Verification items for the finished model (mm, model axes). Round coordinates to 2 decimals unless told otherwise and drop trailing zeros. Write each loop counter-clockwise with the first axis right and the second up, starting at its lowest first coordinate (ties: lowest second). Pieces come first, ordered by that corner, then holes. Notation, with made-up numbers: (-39, 71.25) - (5, 71.25) arc R10 cw to (5, 76.25) - close; hole circle Ø5 at (59, 0.25). An arc over 180 degrees is marked (long way). Answer as a JSON object with one key per item and string values. Group by question number.
1) Section check A-A (x = 27). Enter the section's corners in (y, z) (3 decimals), then the cut area to 3 significant figures.
2) Thickness scan on line 1 (Z direction, x = 36.5, y = 0.25); line 2 (Z direction, x = 5, y = 0.3); line 3 (X direction, y = 0.1, z = -78). Record the ranges inside material, lowest first.
3) Mould release check, pull along Z, two halves, no side actions. Record for faces 1 (the flat face through (20, 0.675, -76)), 2 (the cylindrical face through (3.93, 0.34, -78.54)): +Z half, -Z half, draft (parallel to the pull), parting line (faces both ways), or undercut.
4) Section check C-C (z = -78.5). Enter the section's corners in (x, y) (3 decimals).
5) Section check B-B (y = 0.2). Enter the section's corners in (x, z).
```python
from build123d import *

# Parameters (mm, degrees)
SKETCH1_W           = 35
SKETCH1_H           = 12.964307825
BOSS_EXTRUDE1_DEPTH = 0.675
CUT_EXTRUDE1_DEPTH  = 0.68


with BuildPart() as part:
    # Sketch1 → Boss-Extrude1 (new body)
    with BuildSketch(Plane(origin=(0, 0, 0), x_dir=(1, 0, 0), z_dir=(0, 1, 0))):
        with Locations((19.821319384, 77.80811632)):
            Rectangle(SKETCH1_W, SKETCH1_H)
    extrude(amount=BOSS_EXTRUDE1_DEPTH)

    # Sketch2 → Cut-Extrude1 (cut)
    with BuildSketch(Plane(origin=(0, 0.675, 0), x_dir=(1, 0, 0), z_dir=(0, 1, 0))):
        with BuildLine():
            Line((13.502454123, 76.768011208), (37.321319384, 76.768011208))
            Line((37.321319384, 76.768011208), (37.321319384, 78.518011208))
            Line((37.321319384, 78.518011208), (37.321319384, 80.268011208))
            Line((37.321319384, 80.268011208), (13.502454123, 80.268011208))
            Line((13.502454123, 80.268011208), (4.929914896, 79.518011208))
            ThreePointArc((4.929914896, 79.518011208), (3.929914896, 78.518011208), (4.929914896, 77.518011208))
            Line((4.929914896, 77.518011208), (13.502454123, 76.768011208))
        make_face()
    extrude(amount=-CUT_EXTRUDE1_DEPTH, mode=Mode.SUBTRACT)


solid = part.part
```
Returned:
{
 "1": {"outline": "(0, -84.29) - (0.675, -84.29) - (0.675, -80.268) - (0, -80.268) - close; (0, -76.768) - (0.675, -76.768) - (0.675, -71.326) - (0, -71.326) - close", "area": "6.39 mm2"},
 "2": {"line 1": "-84.29 to -80.27, -76.77 to -71.33", "line 2": "-84.29 to -79.52, -77.51 to -71.33", "line 3": "2.32 to 4.07"},
 "3": {"face 1": "draft", "face 2": "undercut"},
 "4": {"outline": "(2.321, 0) - (3.93, 0) - (3.93, 0.675) - (2.321, 0.675) - close"},
 "5": {"outline": "(2.32, -84.29) - (37.32, -84.29) - (37.32, -80.27) - (13.5, -80.27) - (4.93, -79.52) arc R1 cw to (4.93, -77.52) - (13.5, -76.77) - (37.32, -76.77) - (37.32, -71.33) - (2.32, -71.33) - close"}
}
